Source: CAD feature listing. Evaluate the final solid. Frame: model axes, mm. A direction names the side the tool comes from. Give positions to 0.01 mm unless a question says otherwise; leave off trailing zeros. Loops run counter-clockwise (first coordinate to the right, second up) from the corner with the lowest first, then second, coordinate; pieces in that order, holes last. Notation, with made-up numbers: M -13,42 L -6,42 A22 cw -6,78 Z; hole C -5,84 d3. An arc over 180 degrees is marked long. Answer in a Markdown table with one row per item.
```python
from build123d import *

# Parameters (mm, degrees)
F0_W     = 40
F0_H     = 83
F0_W_2   = 55
F1_DEPTH = 10.31
F2_R     = 5
F3_DEPTH = 10.311
F4_DEPTH = 6


with BuildPart() as f1:
    # F0 (on Top) → F1 (new body)
    with BuildSketch(Plane.XY):
        with Locations((-47.5, 0)):
            Rectangle(F0_W, F0_H)
        Rectangle(F0_W_2, F0_H)
        with Locations((47.5, 0)):
            Rectangle(F0_W, F0_H)
    extrude(amount=-F1_DEPTH)

    # F2 (on face) → F3 (cut, through all)
    with BuildSketch(Plane.XY):
        with Locations((52.5, 26.5)):
            Circle(F2_R)
        with Locations((52.5, -26.5)):
            Circle(F2_R)
        with Locations((-52.5, 26.5)):
            Circle(F2_R)
        with Locations((-52.5, -26.5)):
            Circle(F2_R)
    extrude(amount=-F3_DEPTH, mode=Mode.SUBTRACT)

    # F0 (on Top) → F4 (join)
    with BuildSketch(Plane.XY):
        Rectangle(F0_W_2, F0_H)
    extrude(amount=F4_DEPTH)


solid = f1.part
```
1) Material intervals for L1, parallel to Y at x = 52.5, z = -3.25; L2, parallel to Y at x = -49, z = -3.5; L3, parallel to Z at x = 33.5, y = -15, sorted ascending.
Reply:
| item | result |
|---|---|
| L1 | y = -41.5 to -31.5, -21.5 to 21.5, 31.5 to 41.5 |
| L2 | y = -41.5 to -30.07, -22.93 to 22.93, 30.07 to 41.5 |
| L3 | z = -10.31 to 0 |
2) Pull-direction query (X, two-part tool) for faces 4 (the flat face through (67.5, -1, -5)), 5 (the cylindrical face through (51.42, 21.62, -5.08)), 6 (the flat face through (-1, -41.5, -4)); classes: released by +X, released by -X, zero draft, split by the parting line, or undercut.
Reply:
| item | result |
|---|---|
| face 4 | released by +X |
| face 5 | undercut |
| face 6 | zero draft |
3) Set-up query: faces 1 (the flat face through (27.5, -1, 3)), 2 (the flat face through (-67.5, -1, -5)), 3 (the flat face through (-48, 1, 0)). Return all of +Z, -Z, +X, -X, +Y, -Y with unobstructed straight access to the full face (end or side cutting, diameter ignored); none if empty.
Reply:
| item | result |
|---|---|
| face 1 | +Z, +X, +Y, -Y |
| face 2 | +Z, -Z, -X, +Y, -Y |
| face 3 | +Z, -X, +Y, -Y |
4) Section C-C, the plane z = -3.5. Return loops of the section in (x, y), then the cut area to 3 significant figures.
Reply:
| item | result |
|---|---|
| outline | M -67.5,-41.5 L 67.5,-41.5 L 67.5,41.5 L -67.5,41.5 Z; hole C -52.5,-26.5 d10; hole C -52.5,26.5 d10; hole C 52.5,-26.5 d10; hole C 52.5,26.5 d10 |
| area | 10,900 mm² |
5) Section A-A, the plane y = -26.5. Return loops of the section in (x, z), then the cut area to 3 significant figures.
Reply:
| item | result |
|---|---|
| outline | M -67.5,-10.31 L -57.5,-10.31 L -57.5,0 L -67.5,0 Z; M -47.5,-10.31 L 47.5,-10.31 L 47.5,0 L 27.5,0 L 27.5,6 L -27.5,6 L -27.5,0 L -47.5,0 Z; M 57.5,-10.31 L 67.5,-10.31 L 67.5,0 L 57.5,0 Z |
| area | 1,520 mm² |
6) Section B-B, the plane x = -52.5. Return loops of the section in (y, z), then the cut area to 3 significant figures.
Reply:
| item | result |
|---|---|
| outline | M -41.5,-10.31 L -31.5,-10.31 L -31.5,0 L -41.5,0 Z; M -21.5,-10.31 L 21.5,-10.31 L 21.5,0 L -21.5,0 Z; M 31.5,-10.31 L 41.5,-10.31 L 41.5,0 L 31.5,0 Z |
| area | 650 mm² |
7) Section D-D, the plane y = -35.5. Return loops of the section in (x, z), then the cut area to 3 significant figures.
Reply:
| item | result |
|---|---|
| outline | M -67.5,-10.31 L 67.5,-10.31 L 67.5,0 L 27.5,0 L 27.5,6 L -27.5,6 L -27.5,0 L -67.5,0 Z |
| area | 1,720 mm² |
8) Pin query (flat end, axial travel): pin 1 Ø5 at (y, z) = (-4.5, 4) entering from -X; pin 2 Ø11.5 at (x, y) = (52.5, 26.5) entering from +Z; pin 3 Ø3 at (y, z) = (-6.5, 3) entering from +X. Return the tip coordinate at first contact, or that it passes through.
Reply:
| item | result |
|---|---|
| pin 1 | stops at x = -27.5 |
| pin 2 | stops at z = 0 |
| pin 3 | stops at x = 27.5 |
